Input: dimensioned drawing with shaded views. Units: mm. Origin: part minimum x, y, z. A direction names the side the tool comes from. Coordinates: 2 decimals unless noted, no trailing zeros. Order: outer loops, then holes, each group sorted by start corner. A loop starts at its lowest first (then second) coordinate and runs counter-clockwise, first axis right, second up. Notation, with made-up numbers: (84, -18) -> (100, -18) arc R29 ccw to (100, 6) -> close; hole circle Ø11 at (59.25, 37.5). An arc over 180 degrees is marked (long way). Put each result on its own line as item: value.
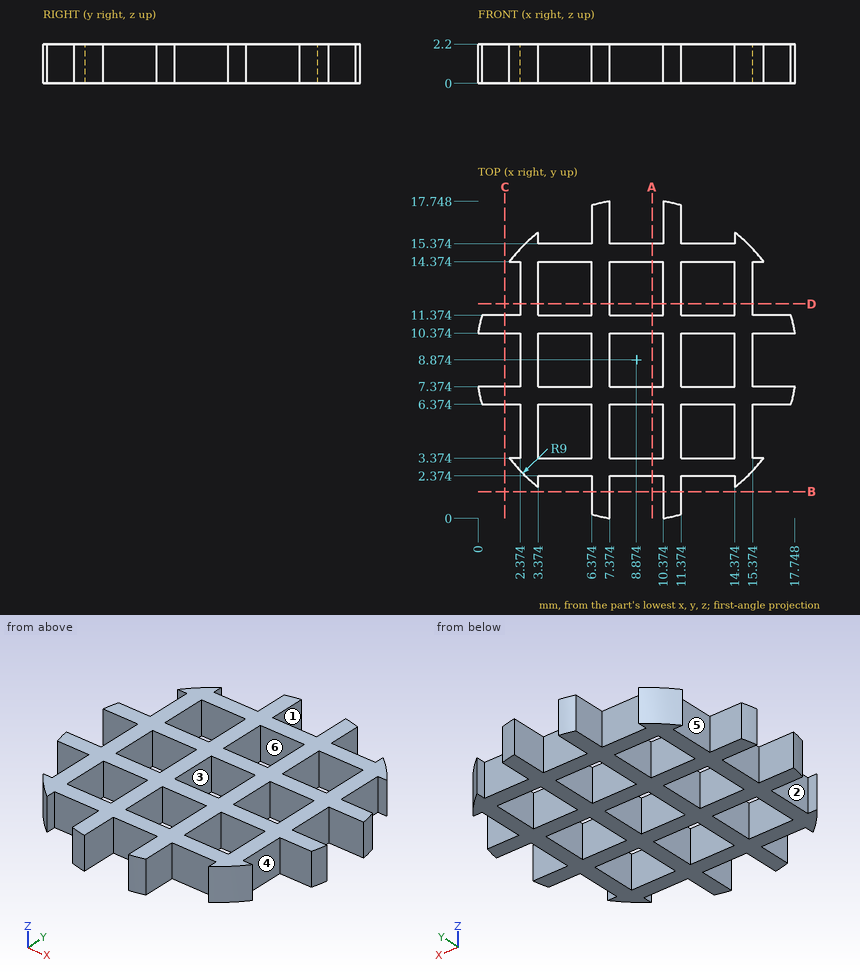
1. Cut plane A-A on x = 9.75. Output: boundary loops of the cut face in (y, z).
Numbers:
outline: (2.37, 0) -> (3.37, 0) -> (3.37, 2.2) -> (2.37, 2.2) -> close; (6.37, 0) -> (7.37, 0) -> (7.37, 2.2) -> (6.37, 2.2) -> close; (10.37, 0) -> (11.37, 0) -> (11.37, 2.2) -> (10.37, 2.2) -> close; (14.37, 0) -> (15.37, 0) -> (15.37, 2.2) -> (14.37, 2.2) -> close
2. Set-up query: the marked faces 1, 2 and 3. Return all of +Z, -Z, +X, -X, +Y, -Y with unobstructed straight access to the full face (end or side cutting, diameter ignored); none if empty.
Numbers:
face 1: +Z, -Z, +Y
face 2: +Z, -Z, -X
face 3: +Z, -Z
3. First-contact query: pin 1 (0.7 mm diameter, centred on x = 1, z = 1.5, fed in from +Y); pin 2 (1.1 mm diameter, centred on x = 13, z = 1, fed in from +Y); pin 3 (1 mm diameter, centred on y = 11, z = 0.5, fed in from -X); pin 4 (5 mm diameter, centred on x = 8.5, y = 11, fed in from -Z). Flat tips, straight axial feed; report the tip coordinate or a pass-through.
Numbers:
pin 1: stops at y = 11.37
pin 2: stops at y = 15.37
pin 3: stops at x = 0.02
pin 4: stops at z = 0
4. Ray query, line 1 along X through (y, z) = (5, 1.8); line 2 along X through (y, z) = (16.75, 1.8). Return the intervals inside material, ascending.
Numbers:
line 1: x = 2.37 to 3.37, 6.37 to 7.37, 10.37 to 11.37, 14.37 to 15.37
line 2: x = 6.37 to 7.37, 10.37 to 11.37
5. Pull-direction query (X, two-part tool) for the marked faces 4, 5 and 6; classes: pulls with the +X half, pulls with the -X half, needs draft (parallel to the pull), parting line crosses it, or undercut.
Numbers:
face 4: pulls with the +X half
face 5: pulls with the -X half
face 6: undercut
6. Cut plane B-B on y = 1.5. Output: boundary loops of the cut face in (x, z).
Numbers:
outline: (6.37, 0) -> (7.37, 0) -> (7.37, 2.2) -> (6.37, 2.2) -> close; (10.37, 0) -> (11.37, 0) -> (11.37, 2.2) -> (10.37, 2.2) -> close
